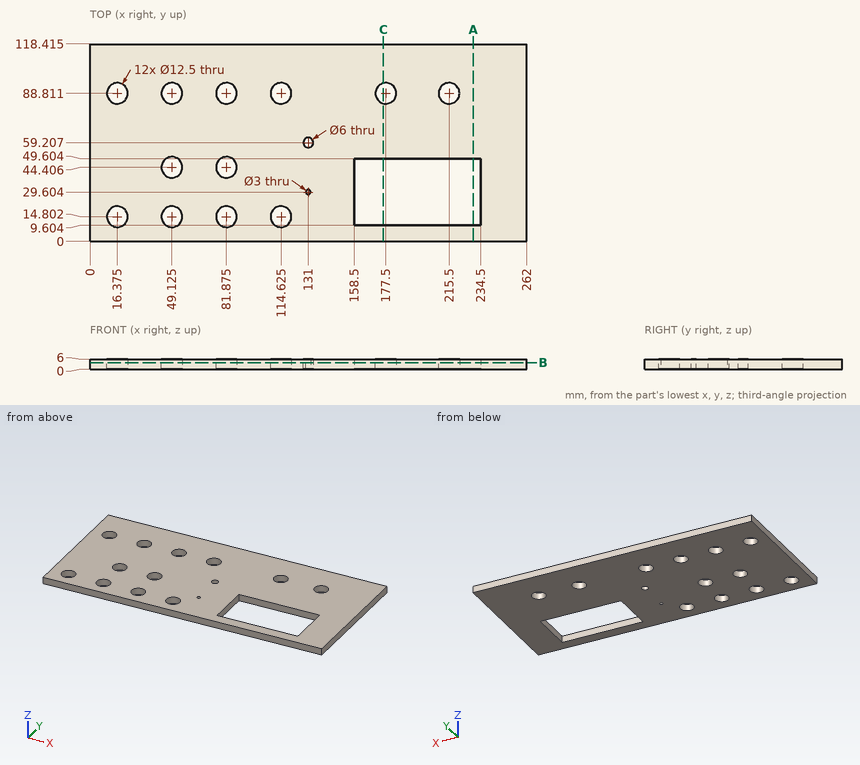
Here's the drawing with two shaded views (mm, measured from the low corner). I have some questions. Round coordinates to 2 decimals unless told otherwise and drop trailing zeros. Loops run counter-clockwise (first coordinate to the right, second up) from the corner with the lowest first, then second, coordinate; pieces in that order, holes last.
1. Suppose I cut it at C-C, the plane x = 176. Please give me the cut outline in (y, z) (1 decimal).
Answers:
outline: (0, 0) - (9.6, 0) - (9.6, 6) - (0, 6) - close; (49.6, 0) - (82.7, 0) - (82.7, 6) - (49.6, 6) - close; (94.9, 0) - (118.4, 0) - (118.4, 6) - (94.9, 6) - close
2. If I drill on probe 1 along Y at (x, z) = (131, 1.45) (1 decimal); probe 2 along Y at (x, z) = (206, 4.55) (1 decimal); probe 3 along X at (y, z) = (44.5, 1.65) (1 decimal), over which ranges is the centre line in solid material (lowest first)?
Answers:
probe 1: y = 0 to 28.1, 31.1 to 56.2, 62.2 to 118.4
probe 2: y = 0 to 9.6, 49.6 to 118.4
probe 3: x = 0 to 42.9, 55.4 to 75.6, 88.1 to 158.5, 234.5 to 262
3. Suppose I cut it at A-A, the plane x = 230. Please give me the cut outline in (y, z) (1 decimal).
Answers:
outline: (0, 0) - (9.6, 0) - (9.6, 6) - (0, 6) - close; (49.6, 0) - (118.4, 0) - (118.4, 6) - (49.6, 6) - close
4. Will this pin go through, and if not, where does the flat tip stop? pin 1 (2 mm diameter, centred on x = 164, y = 48, fed in from -Z) (3 decimals).
Answers:
pin 1: passes through
5. Suppose I cut it at B-B, the plane z = 4.1. Give the number of separate pieces and of enclosed holes in the cut face, and give its area (3 significant figures).
Answers:
separate pieces: 1
enclosed holes: 15
area: 26,500 mm2
